CAD build for the part. Positions are in the model's coordinates, mm. Coordinates: 2 decimals unless noted, no trailing zeros. Loops run counter-clockwise (first coordinate to the right, second up) from the corner with the lowest first, then second, coordinate; pieces in that order, holes last.
1) Pin check, flat tips, straight feed: pin 1 Ø8 at (x, y) = (17, 4) entering from +Z; pin 2 Ø4 at (y, z) = (4, 60) entering from +X; pin 3 Ø1.5 at (y, z) = (1, 48) entering from -X. Stop position of each tip, or through.
2) Saw through at A-A, the plane y = -5.5. Write the cut outline in (x, z), and give its area (3 significant figures).
3) Wall check: line 1 along Z through (x, y) = (28.5, 12); line 2 along X through (y, z) = (7.5, 73); line 3 along Z through (x, y) = (-36, -8). Give the ranges that are in metal, low to high.
4) Saw through at B-B, the plane y = -21. Write the cut outline in (x, z).
```python
from build123d import *

# Parameters (mm, degrees)
CYLINDER030_R          = 100
CYLINDER030_DEPTH      = 86
CYLINDER030_ROLL_ANGLE = 90
CYLINDER_R             = 50
CYLINDER_DEPTH         = 70
CYLINDER_ROLL_ANGLE    = 90
TORUS_R                = 35
TORUS_ROLL_ANGLE       = 90
CYLINDER029_R          = 60
CYLINDER029_DEPTH      = 86
CYLINDER029_ROLL_ANGLE = 90
TORUS001_R             = 36
TORUS001_ROLL_ANGLE    = 90


with BuildPart() as cilindro030:
    # Cylinder030 → Cylinder030 (new body)
    with BuildSketch(Plane.XY):
        Circle(CYLINDER030_R)
    extrude(amount=CYLINDER030_DEPTH)


with BuildPart() as cilindro030_1:
    # Cylinder030 roll: moved
    add(cilindro030.part.rotate(Axis((0, 0, 0), (1, 0, 0)), CYLINDER030_ROLL_ANGLE))


with BuildPart() as cilindro030_2:
    # Cylinder030 placement: moved
    add(cilindro030_1.part.moved(Location((0, -30, 0))))


with BuildPart() as fusion021:
    # Part__Mirroring005: instance of Cilindro030
    add(cilindro030_2.part.mirror(Plane(origin=(0, 0, 0), x_dir=(1, 0, 0), z_dir=(0, 1, 0))))

    # Fusion021: union Cilindro030
    add(cilindro030_2.part)


with BuildPart() as cilindro:
    # Cylinder → Cylinder (new body)
    with BuildSketch(Plane.XY):
        Circle(CYLINDER_R)
    extrude(amount=CYLINDER_DEPTH)


with BuildPart() as cilindro_1:
    # Cylinder roll: moved
    add(cilindro.part.rotate(Axis((0, 0, 0), (1, 0, 0)), CYLINDER_ROLL_ANGLE))


with BuildPart() as cilindro_2:
    # Cylinder placement: moved
    add(cilindro_1.part.moved(Location((0, 35, 0))))


with BuildPart() as clone_of_fusion:
    # Torus → Torus (revolve)
    with BuildSketch(Plane.XZ):
        with Locations((50, 0)):
            Circle(TORUS_R)
    revolve(axis=Axis((0, 0, 0), (0, 0, 1)))


with BuildPart() as clone_of_fusion_1:
    # Torus roll: moved
    add(clone_of_fusion.part.rotate(Axis((0, 0, 0), (1, 0, 0)), TORUS_ROLL_ANGLE))


with BuildPart() as clone_of_fusion_2:
    # Torus placement: moved
    add(clone_of_fusion_1.part)

    # Fusion: union Cilindro
    add(cilindro_2.part)


with BuildPart() as cilindro029:
    # Cylinder029 → Cylinder029 (new body)
    with BuildSketch(Plane.XY):
        Circle(CYLINDER029_R)
    extrude(amount=CYLINDER029_DEPTH)


with BuildPart() as cilindro029_1:
    # Cylinder029 roll: moved
    add(cilindro029.part.rotate(Axis((0, 0, 0), (1, 0, 0)), CYLINDER029_ROLL_ANGLE))


with BuildPart() as cilindro029_2:
    # Cylinder029 placement: moved
    add(cilindro029_1.part.moved(Location((0, 42, 0))))


with BuildPart() as cut030:
    # Torus001 → Torus001 (revolve)
    with BuildSketch(Plane.XZ):
        with Locations((50, 0)):
            Circle(TORUS001_R)
    revolve(axis=Axis((0, 0, 0), (0, 0, 1)))


with BuildPart() as cut030_1:
    # Torus001 roll: moved
    add(cut030.part.rotate(Axis((0, 0, 0), (1, 0, 0)), TORUS001_ROLL_ANGLE))


with BuildPart() as cut030_2:
    # Torus001 placement: moved
    add(cut030_1.part)

    # Cut028: cut Cilindro029
    add(cilindro029_2.part, mode=Mode.SUBTRACT)

    # Cut029: cut Clone of Fusion
    add(clone_of_fusion_2.part, mode=Mode.SUBTRACT)

    # Cut030: cut Fusion021
    add(fusion021.part, mode=Mode.SUBTRACT)


solid = cut030_2.part
```
Data:
1. pin 1: stops at z = 84.88
1. pin 2: stops at x = 63.22
1. pin 3: stops at x = -71.84
2. outline: circle Ø171.15 at (0, 0); hole circle Ø169.13 at (0, 0)
2. area: 541 mm2
3. line 1: z = -78.95 to -77.82, 77.82 to 78.95
3. line 2: x = -43.95 to -41.93, 41.93 to 43.95
3. line 3: z = -77.11 to -75.98, 75.98 to 77.11
4. outline: circle Ø158.48 at (0, 0); hole circle Ø156 at (0, 0)
